Verification items for the finished model (mm, model axes). Face numbers are marked on the shaded views. Round coordinates to 2 decimals unless told otherwise and drop trailing zeros. Write each loop counter-clockwise with the first axis right and the second up, starting at its lowest first coordinate (ties: lowest second). Pieces come first, ordered by that corner, then holes. Notation, with made-up numbers: (29.5, 86) -> (86.5, 86) arc R27 ccw to (86.5, 106) -> close; hole circle Ø5 at (-4, 60.5). An arc over 180 degrees is marked (long way). Answer as a JSON object with one key per item and string values. Group by question number.
(1) Sectioned sample at B-B on x = 70. Record the cut outline in (y, z), and give its area (3 significant figures).
(2) Gauge pin test, flat ends, axial feed: pin 1 Ø8 at (x, z) = (11, -70.5) entering from -Y; pin 2 Ø5 at (x, z) = (11.5, -10.5) entering from -Y; pin 3 Ø3 at (y, z) = (1.5, -56) entering from +X. Record the tip position at first contact, or that the pin passes through.
(3) Sectioned sample at A-A on z = -90. Record the cut outline in (x, y).
(4) Scan lines: L1, parallel to Z at x = 110, y = 0.85; L2, parallel to Z at x = 110, y = 4.15; L3, parallel to X at y = 1, z = -94.5. Record each from-to range of solid material in increasing order. Write a range as from..to.
(5) Draft check along Y on the marked faces 1 and 2. Enter one of: released by +Y, released by -Y, zero draft, split by the parting line, or undercut.
(6) Sectioned sample at C-C on x = 10. Count the separate pieces of the cut face and the enclosed holes in it, and give its area (3 significant figures).
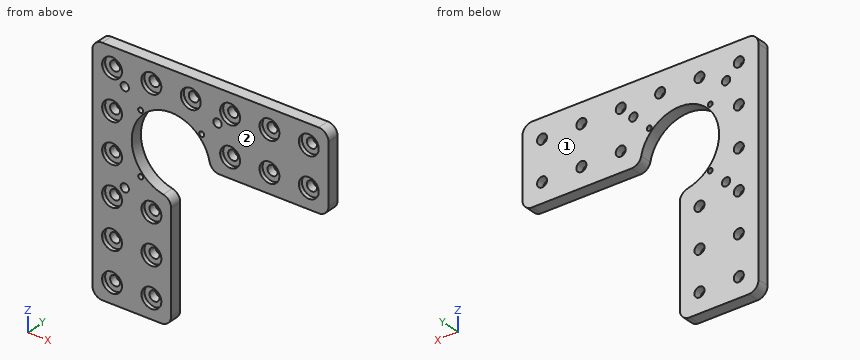
```python
from build123d import *

# Parameters (mm, degrees)
F1_DEPTH       = 6
F2_D           = 5.1
F2_CBORE_D     = 10.1
F2_CBORE_DEPTH = 2
F3_D           = 4.2
F4_D           = 2.5


with BuildPart() as f1:
    # F0 (on Front) → F1 (new body)
    with BuildSketch(Plane.XZ):
        with BuildLine():
            Line((115, 0), (5, 0))
            ThreePointArc((5, 0), (1.4644660941, -1.4644660941), (0, -5))
            Line((0, -5), (0, -115))
            ThreePointArc((0, -115), (1.4644660941, -118.5355339059), (5, -120))
            Line((5, -120), (35, -120))
            ThreePointArc((35, -120), (38.5355339059, -118.5355339059), (40, -115))
            Line((40, -115), (40, -64.4948974278))
            ThreePointArc((40, -64.4948974278), (38.8729833462, -61.3326197677), (36, -59.5959179423))
            ThreePointArc((36, -59.5959179423), (25.8578643763, -25.8578643763), (59.5959179423, -36))
            ThreePointArc((59.5959179423, -36), (61.3326197677, -38.8729833462), (64.4948974278, -40))
            Line((64.4948974278, -40), (115, -40))
            ThreePointArc((115, -40), (118.5355339059, -38.5355339059), (120, -35))
            Line((120, -35), (120, -5))
            ThreePointArc((120, -5), (118.5355339059, -1.4644660941), (115, 0))
        make_face()
    extrude(amount=-F1_DEPTH)

    # F2 (through all)
    with Locations(Plane.XZ):
        with Locations((10, -110), (30, -110), (30, -90), (10, -90), (10, -70), (30, -70), (10, -50), (10, -30), (10, -10), (30, -10), (50, -10), (70, -10), (70, -30), (90, -30), (90, -10), (110, -10), (110, -30)):
            CounterBoreHole(F2_D / 2, F2_CBORE_D / 2, F2_CBORE_DEPTH)

    # F3 (through all)
    with Locations(Plane.XZ):
        with Locations((16.468, -16.392), (63.6079993896, -16.392), (16.468, -63.5319993896)):
            Hole(F3_D / 2)

    # F4 (through all)
    with Locations(Plane.XZ):
        with Locations((24.538, -24.462), (55.538, -24.462), (24.538, -55.462)):
            Hole(F4_D / 2)


solid = f1.part
```
Computed values:
{
 "1": {"outline": "(0, -40) -> (6, -40) -> (6, -32.55) -> (2, -32.55) -> (2, -35.05) -> (0, -35.05) -> close; (0, -24.95) -> (2, -24.95) -> (2, -27.45) -> (6, -27.45) -> (6, -12.55) -> (2, -12.55) -> (2, -15.05) -> (0, -15.05) -> close; (0, -4.95) -> (2, -4.95) -> (2, -7.45) -> (6, -7.45) -> (6, 0) -> (0, 0) -> close", "area": "159 mm2"},
 "2": {"pin 1": "y = 0", "pin 2": "y = 2", "pin 3": "x = 30.32"},
 "3": {"outline": "(0, 0) -> (4.95, 0) -> (4.95, 2) -> (7.45, 2) -> (7.45, 6) -> (0, 6) -> close; (12.55, 2) -> (15.05, 2) -> (15.05, 0) -> (24.95, 0) -> (24.95, 2) -> (27.45, 2) -> (27.45, 6) -> (12.55, 6) -> close; (32.55, 2) -> (35.05, 2) -> (35.05, 0) -> (40, 0) -> (40, 6) -> (32.55, 6) -> close"},
 "4": {"L1": "-40..-35.05, -24.95..-15.05, -4.95..0", "L2": "-40..-32.55, -27.45..-12.55, -7.45..0", "L3": "0..7.71, 12.29..27.71, 32.29..40"},
 "5": {"face 1": "released by +Y", "face 2": "released by -Y"},
 "6": {"separate pieces": "7", "enclosed holes": "0", "area": "476 mm2"}
}
